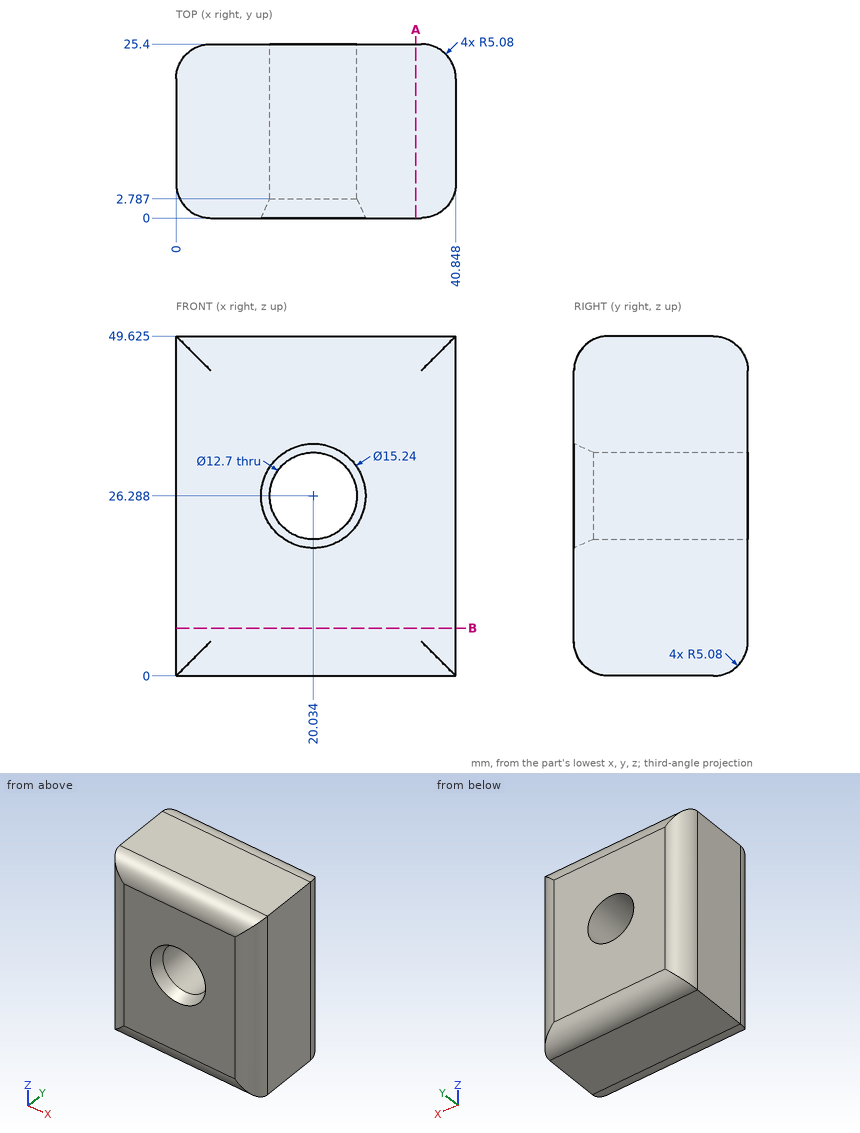
Print and shaded views of the part. All mm, measured from the part's lowest x, y and z. Round coordinates to 2 decimals unless told otherwise and drop trailing zeros. Write each loop counter-clockwise with the first axis right and the second up, starting at its lowest first coordinate (ties: lowest second). Pieces come first, ordered by that corner, then holes. Notation, with made-up numbers: (-31, -11) -> (-1, -11) arc R20 ccw to (-1, 2) -> close; hole circle Ø8 at (28.5, 81). An arc over 180 degrees is marked (long way). Return JSON: item names as keys, results as strings. Group by question number.
Q1. Saw through at A-A on x = 35. Write the cut outline in (y, z) (1 decimal).
Q2. Saw through at B-B on z = 7. Write the cut outline in (x, y), plus the area to 3 significant figures.
Q3. Probe L1, parallel to X at y = 11.75, z = 26.5; L2, parallel to Z at x = 17.5, y = 23 (1 decimal); L3, parallel to Z at x = 23, y = 12.75 (1 decimal). List the from-to ranges inside material, lowest first. Write a range as [from, to].
Answer:
{
 "1": {"outline": "(0, 5.1) arc R5.1 ccw to (5.1, 0) -> (20.3, 0) arc R5.1 ccw to (25.4, 5.1) -> (25.4, 44.5) arc R5.1 ccw to (20.3, 49.6) -> (5.1, 49.6) arc R5.1 ccw to (0, 44.5) -> close"},
 "2": {"outline": "(0, 5.08) arc R5.08 ccw to (5.08, 0) -> (35.77, 0) arc R5.08 ccw to (40.85, 5.08) -> (40.85, 20.32) arc R5.08 ccw to (35.77, 25.4) -> (5.08, 25.4) arc R5.08 ccw to (0, 20.32) -> close", "area": "1,020 mm2"},
 "3": {"L1": "[0, 13.69], [26.38, 40.85]", "L2": "[0.8, 20.5], [32.1, 48.9]", "L3": "[0, 20.7], [31.9, 49.6]"}
}
